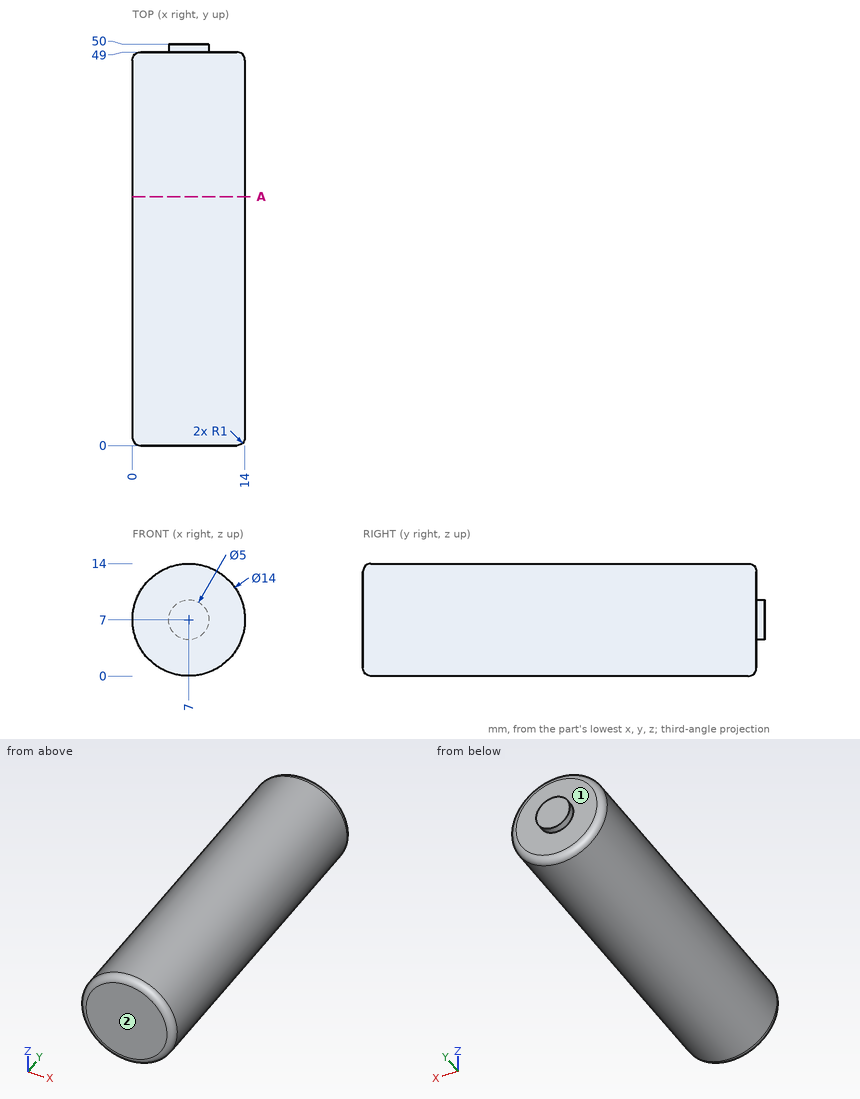
Here's the drawing with two shaded views (mm, measured from the low corner). I have some questions. A direction names the side the tool comes from. Give positions to 0.01 mm unless a question says otherwise; leave off trailing zeros. Order: outer loops, then holes, each group sorted by start corner. A loop starts at its lowest first (then second) coordinate and runs counter-clockwise, first axis right, second up. Notation, with made-up numbers: M 52,0.5 L 111,0.5 A26 ccw 111,21.5 Z; hole C -0.75,40 d4. An arc over 180 degrees is marked long. Answer as a JSON object with one key per item and string values. Group by question number.
1) I'm going to push flat-ended pins straight in: pin 1 Ø3 at (x, y) = (10.5, 37.5) entering from -Z; pin 2 Ø5 at (y, z) = (18.5, 3.5) entering from +X; pin 3 Ø1.5 at (y, z) = (16.5, 11) entering from +X. Where does each tip first touch, or does it pass through?
2) On a 3-axis mill with a long thin cutter (end or side, diameter ignored), from which of +Z, -Z, +X, -X, +Y, -Y can I reach the whole of each face in a straight line? I mean the marked faces 1 and 2. Say none if no direction works.
3) Please list where these lines run through material, in increasing order: L1, parallel to Y at x = 7.5, z = 11; L2, parallel to Z at x = 7.25, y = 14.5; L3, parallel to X at y = 35.5, z = 5.5. Write a range as [from, to].
4) Suppose I cut it at A-A, the plane y = 31. Write out the boundary of the cut face in (x, z), plus the area to 3 significant figures.
Results found:
{
 "1": {"pin 1": "z = 0.29", "pin 2": "x = 13.93", "pin 3": "x = 13.2"},
 "2": {"face 1": "+Y", "face 2": "+Z, -Z, +X, -X, -Y"},
 "3": {"L1": "[0, 49]", "L2": "[0, 14]", "L3": "[0.16, 13.84]"},
 "4": {"outline": "C 7,7 d14", "area": "154 mm²"}
}
